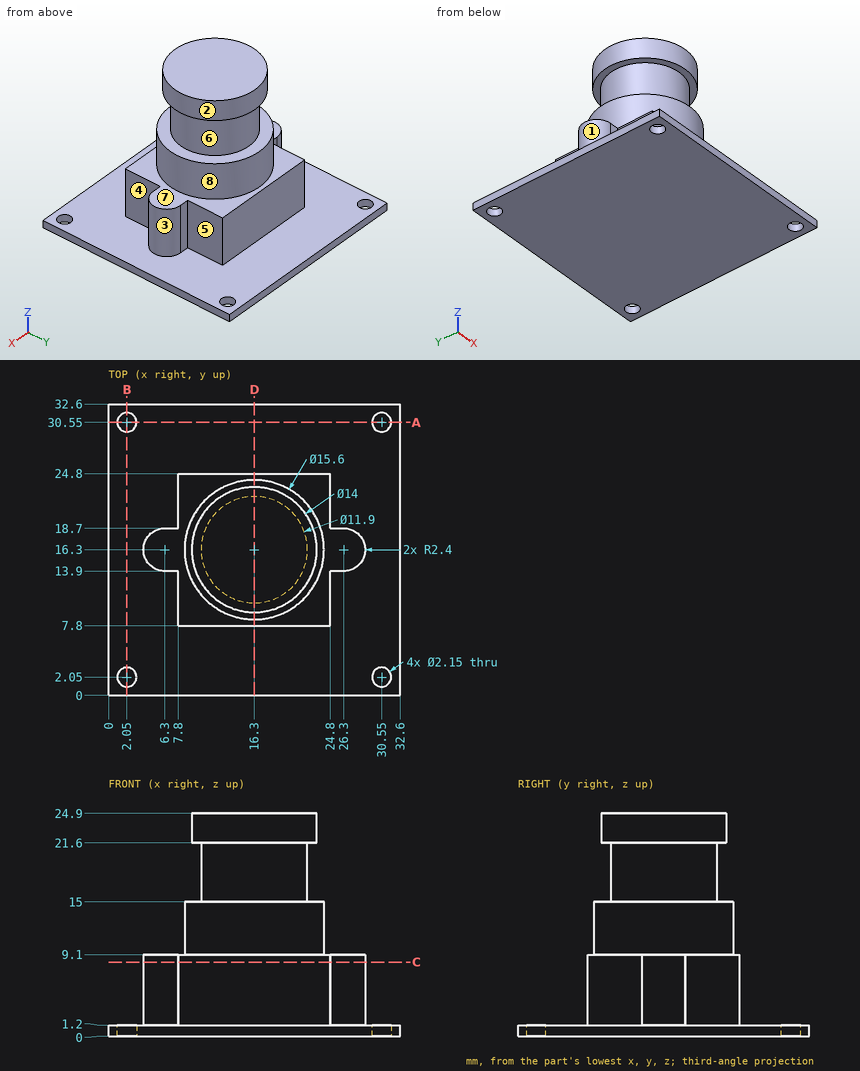
For this review, use the dimensioned drawing (mm, ordinates from the lowest corner) and the shaded views. A direction names the side the tool comes from. Coordinates: 2 decimals unless noted, no trailing zeros. Loops run counter-clockwise (first coordinate to the right, second up) from the corner with the lowest first, then second, coordinate; pieces in that order, holes last.
1. For line 1 (Y direction, x = 2.05, z = 0.7) (3 decimals); line 2 (Z direction, x = 10, y = 16.5); line 3 (Z direction, x = 31, y = 3.5), list the stretches that pass through material, from the lowest coordinate up.
2. Add section D-D, the plane x = 16.3. Give the boundary of the cut face in (y, z).
3. Add section C-C, the plane z = 8.25. Give the boundary of the cut face in (x, y).
4. Add section A-A, the plane y = 30.55. Give the boundary of the cut face in (x, z) (3 decimals).
5. Insertion check: P1, Ø12, axis at x = 6, z = 10.5, coming from the +Y side; P2, Ø5, axis at x = 28, y = 24.5, coming from the +Z side; P3, Ø2, axis at y = 20, z = 5.5, coming from the +X side; P4, Ø1.5, axis at y = 27.5, z = 4, coming from the -X side. Each pin has a flat end and moves straight along its axis. Give the tip position at first contact, or say it passes through.
6. For the marked faces 1, 2, 3, 4 and 5, list the 3-axis set-ups (+Z, -Z, +X, -X, +Y, -Y) from which the entire face can be reached by the end or side of a thin tool; tool diameter is ignored.
7. Mouldability with a two-part tool opening along Z and no side actions: class the marked faces 6, 7 and 8 as +Z half, -Z half, draft (parallel to the pull), parting line (faces both ways), or undercut.
Result:
1. line 1: y = 0 to 0.975, 3.125 to 29.475, 31.625 to 32.6
1. line 2: z = 0 to 15, 21.6 to 24.9
1. line 3: z = 0 to 1.2
2. outline: (0, 0) - (32.6, 0) - (32.6, 1.2) - (24.8, 1.2) - (24.8, 9.1) - (24.1, 9.1) - (24.1, 15) - (22.25, 15) - (22.25, 21.6) - (23.3, 21.6) - (23.3, 24.9) - (9.3, 24.9) - (9.3, 21.6) - (10.35, 21.6) - (10.35, 15) - (8.5, 15) - (8.5, 9.1) - (7.8, 9.1) - (7.8, 1.2) - (0, 1.2) - close
3. outline: (6.3, 13.9) - (7.8, 13.9) - (7.8, 7.8) - (24.8, 7.8) - (24.8, 13.9) - (26.3, 13.9) arc R2.4 ccw to (26.3, 18.7) - (24.8, 18.7) - (24.8, 24.8) - (7.8, 24.8) - (7.8, 18.7) - (6.3, 18.7) arc R2.4 ccw to start
4. outline: (0, 0) - (0.975, 0) - (0.975, 1.2) - (0, 1.2) - close; (3.125, 0) - (29.475, 0) - (29.475, 1.2) - (3.125, 1.2) - close; (31.625, 0) - (32.6, 0) - (32.6, 1.2) - (31.625, 1.2) - close
5. P1: stops at y = 24.8
5. P2: stops at z = 1.2
5. P3: stops at x = 24.8
5. P4: passes through
6. face 1: +Z, -X
6. face 2: +Z
6. face 3: +Z, +X
6. face 4: +Z, +X, -Y
6. face 5: +Z, +X, +Y
7. face 6: undercut
7. face 7: +Z half
7. face 8: draft
